Read the model definition and answer for the solid it produces. Units are mm, in the model's axes. Face numbers are marked on the shaded views. Give positions to 0.01 mm unless a question says otherwise; leave off trailing zeros. Write each loop counter-clockwise with the first axis right and the second up, starting at its lowest first coordinate (ties: lowest second). Pieces come first, ordered by that corner, then holes.
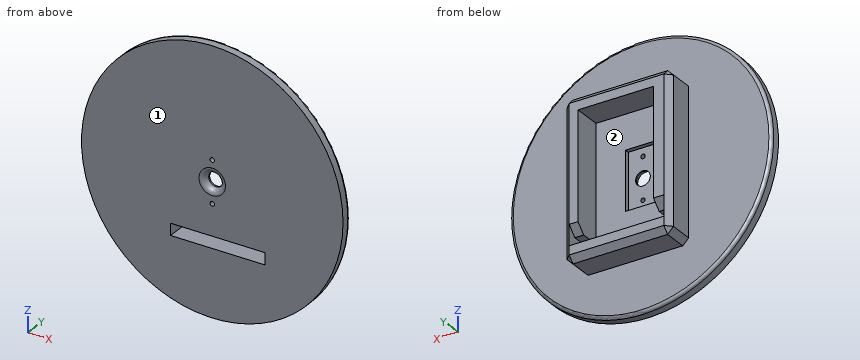
```python
from build123d import *

# Parameters (mm, degrees)
SKETCH1_R           = 44.45
BOSS_EXTRUDE1_DEPTH = 3.5
CUT_EXTRUDE1_DEPTH  = 1
SKETCH3_W           = 25.675
SKETCH3_H           = 43.475
BOSS_EXTRUDE2_DEPTH = 10
SKETCH4_W           = 25.675
SKETCH4_H           = 4
CUT_EXTRUDE2_DEPTH  = 13
SKETCH5_R           = 0.75
CUT_EXTRUDE3_DEPTH  = 13
SKETCH6_R           = 2.5
CUT_EXTRUDE4_DEPTH  = 13
FILLET1_R           = 1
CHAMFER1_SIZE       = 2
FILLET2_R           = 2
SKETCH8_W           = 3.5
SKETCH8_H           = 4
CUT_EXTRUDE6_DEPTH  = 14.5000001
SKETCH10_W          = 3
SKETCH10_H          = 4
CUT_EXTRUDE7_DEPTH  = 14.5000001
CHAMFER2_SIZE       = 3
SKETCH11_W          = 25.675
SKETCH11_H          = 39.475
BOSS_EXTRUDE3_DEPTH = 1.5


with BuildPart() as part:
    # Sketch1 → Boss-Extrude1 (new body)
    with BuildSketch(Plane(origin=(0, 0, 0), x_dir=(1, 0, 0), z_dir=(0, 1, 0))):
        Circle(SKETCH1_R)
    extrude(amount=BOSS_EXTRUDE1_DEPTH)

    # Sketch2 → Cut-Extrude1 (cut)
    with BuildSketch(Plane(origin=(0, 3.5, 0), x_dir=(1, 0, 0), z_dir=(0, 1, 0))):
        Polygon((15, 0), (15, -21.7375), (-10.675, -21.7375), (-10.675, 21.7375), (15, 21.7375), align=None)
    extrude(amount=-CUT_EXTRUDE1_DEPTH, mode=Mode.SUBTRACT)

    # Sketch3 → Boss-Extrude2 (add)
    with BuildSketch(Plane(origin=(0, 3.5, 0), x_dir=(1, 0, 0), z_dir=(0, 1, 0))):
        Polygon((20, -26.7375), (15, -26.7375), (-16.175, -26.7375), (-16.175, 26.7375), (20, 26.7375), align=None)
        with Locations((2.1625, 0)):
            Rectangle(SKETCH3_W, SKETCH3_H, mode=Mode.SUBTRACT)
    extrude(amount=BOSS_EXTRUDE2_DEPTH)

    # Sketch4 → Cut-Extrude2 (cut)
    with BuildSketch(Plane(origin=(0, 2.5, 0), x_dir=(1, 0, 0), z_dir=(0, 1, 0))):
        with Locations((2.1625, 19.7375)):
            Rectangle(SKETCH4_W, SKETCH4_H)
    extrude(amount=-CUT_EXTRUDE2_DEPTH, mode=Mode.SUBTRACT)

    # Sketch5 → Cut-Extrude3 (cut)
    with BuildSketch(Plane(origin=(0, 2.5, 0), x_dir=(1, 0, 0), z_dir=(0, 1, 0))):
        with Locations((0, -7.15)):
            Circle(SKETCH5_R)
        with Locations((0, 7.15)):
            Circle(SKETCH5_R)
    extrude(amount=-CUT_EXTRUDE3_DEPTH, mode=Mode.SUBTRACT)

    # Sketch6 → Cut-Extrude4 (cut)
    with BuildSketch(Plane.XZ):
        Circle(SKETCH6_R)
    extrude(amount=-CUT_EXTRUDE4_DEPTH, mode=Mode.SUBTRACT)

    # Fillet1
    fillet1_edges = [part.edges().sort_by_distance(p)[0] for p in [
        (-44.45, 3.5, 0),
    ]]
    fillet(fillet1_edges, radius=FILLET1_R)

    # Chamfer1
    chamfer1_edges = [part.edges().sort_by_distance(p)[0] for p in [
        (1.9125, 13.5, 26.7375),
        (-16.175, 8.5, 26.7375),
        (20, 13.5, 0),
        (20, 8.5, 26.7375),
        (1.9125, 13.5, -26.7375),
        (20, 8.5, -26.7375),
        (-16.175, 13.5, 0),
        (-16.175, 8.5, -26.7375),
    ]]
    chamfer(chamfer1_edges, length=CHAMFER1_SIZE)

    # Fillet2
    fillet2_edges = [part.edges().sort_by_distance(p)[0] for p in [
        (-2.5, 0, 0),
    ]]
    fillet(fillet2_edges, radius=FILLET2_R)

    # Sketch8 → Cut-Extrude6 (cut, through all)
    with BuildSketch(Plane(origin=(0, 13.5, 0), x_dir=(1, 0, 0), z_dir=(0, 1, 0))):
        with Locations((-12.425, 19.7375)):
            Rectangle(SKETCH8_W, SKETCH8_H)
    extrude(amount=-CUT_EXTRUDE6_DEPTH, mode=Mode.SUBTRACT)

    # Sketch10 → Cut-Extrude7 (cut, through all)
    with BuildSketch(Plane(origin=(0, 13.5, 0), x_dir=(1, 0, 0), z_dir=(0, 1, 0))):
        with Locations((16.5, 19.7375)):
            Rectangle(SKETCH10_W, SKETCH10_H)
    extrude(amount=-CUT_EXTRUDE7_DEPTH, mode=Mode.SUBTRACT)

    # Chamfer2
    chamfer2_edges = [part.edges().sort_by_distance(p)[0] for p in [
        (-12.425, 13.5, -17.7375),
        (16.5, 13.5, -17.7375),
    ]]
    chamfer(chamfer2_edges, length=CHAMFER2_SIZE)

    # Sketch11 → Boss-Extrude3 (add)
    with BuildSketch(Plane(origin=(0, 2.5, 0), x_dir=(1, 0, 0), z_dir=(0, 1, 0))):
        with Locations((2.1625, -2)):
            Rectangle(SKETCH11_W, SKETCH11_H)
        Polygon((-5, 10), (5, 10), (5, 0), (5, -10), (-5, -10), align=None, mode=Mode.SUBTRACT)
    extrude(amount=BOSS_EXTRUDE3_DEPTH)


solid = part.part
```
Item 1: Find the intervals of material crossed by line 1 along Z through (x, y) = (0, 2.3); line 2 along X through (y, z) = (4.75, 9) (3 decimals); line 3 along Z through (x, y) = (0, 1.05), in increasing order.
Result set:
line 1: z = -44.45 to -21.74, -17.74 to -7.9, -6.4 to -2.5, 2.5 to 6.4, 7.9 to 44.45
line 2: x = -16.175 to -10.675, 15 to 20
line 3: z = -44.45 to -21.74, -17.74 to -7.9, -6.4 to -2.74, 2.74 to 6.4, 7.9 to 44.45
Item 2: Each of these flat-tipped pins is pushed along its axis until it touches: pin 1 Ø3 at (x, z) = (-31.5, -26) entering from +Y; pin 2 Ø1 at (y, z) = (10.5, -11) entering from +X; pin 3 Ø5 at (y, z) = (5.5, -14.5) entering from +X; pin 4 Ø8 at (y, z) = (12, -32.5) entering from +X. Where does it stop, or does it pass through?
Result set:
pin 1: stops at y = 3.5
pin 2: stops at x = 20
pin 3: stops at x = 42.05
pin 4: passes through
Item 3: Section B-B (y = 8.5) is taken. Write down the section's boundary in (x, z) (1 decimal).
Result set:
outline: (-16.2, -24.7) - (-14.2, -26.7) - (18, -26.7) - (20, -24.7) - (20, 24.7) - (18, 26.7) - (-14.2, 26.7) - (-16.2, 24.7) - close; hole (-14.2, -21.7) - (18, -21.7) - (18, -17.7) - (15, -17.7) - (15, 21.7) - (-10.7, 21.7) - (-10.7, -17.7) - (-14.2, -17.7) - close
Item 4: Section A-A (z = 0) is taken. Write down the section's boundary in (x, y) (3 decimals), and give its area (3 significant figures).
Result set:
outline: (-44.45, 0) - (-4.5, 0) arc R2 ccw to (-2.5, 2) - (-2.5, 2.5) - (-5, 2.5) - (-5, 4) - (-10.675, 4) - (-10.675, 13.5) - (-14.175, 13.5) - (-16.175, 11.5) - (-16.175, 3.5) - (-43.45, 3.5) arc R1 ccw to (-44.45, 2.5) - close; (2.5, 2) arc R2 ccw to (4.5, 0) - (44.45, 0) - (44.45, 2.5) arc R1 ccw to (43.45, 3.5) - (20, 3.5) - (20, 11.5) - (18, 13.5) - (15, 13.5) - (15, 4) - (5, 4) - (5, 2.5) - (2.5, 2.5) - close
area: 395 mm2
Item 5: Determine the mould class of the marked faces 1 and 2 for opening direction Z: pulls with the +Z half, pulls with the -Z half, needs draft (parallel to the pull), parting line crosses it, or undercut.
Result set:
face 1: needs draft
face 2: undercut
